Check sheet for the modelled part. Datum: model origin and axes. Units: mm. Coordinates: 2 decimals unless noted, no trailing zeros. Loops run counter-clockwise (first coordinate to the right, second up) from the corner with the lowest first, then second, coordinate; pieces in that order, holes last. Notation, with made-up numbers: (87.25, -1) - (91.25, -1) arc R6 cw to (91.25, 10) - close; hole circle Ø7 at (-22.5, -34.75). An arc over 180 degrees is marked (long way). Answer as a JSON object with one key per item and string values. Group by question number.
from build123d import *

# Parameters (mm, degrees)
RESSALTO_EXTRUS_O1_DEPTH = 2
CORTE_EXTRUS_O1_DEPTH    = 3


with BuildPart() as part:
    # Esboço1 → Ressalto-extrusão1 (new body)
    with BuildSketch(Plane(origin=(0, 0, 0), x_dir=(1, 0, 0), z_dir=(0, 1, 0))):
        with BuildLine():
            Line((-65, 27.690493718), (-17.774626759, 33.612777476))
            ThreePointArc((-17.774626759, 33.612777476), (-17.153688565, 33.671045747), (-16.530325742, 33.690493718))
            Line((-16.530325742, 33.690493718), (0, 33.690493718))
            Line((0, 33.690493718), (0, -23.309506282))
            Line((0, -23.309506282), (-24.541301383, -23.309506282))
            ThreePointArc((-24.541301383, -23.309506282), (-27.628384162, -22.821073972), (-30.413900746, -21.403490265))
            Line((-30.413900746, -21.403490265), (-65, 3.690493718))
            Line((-65, 3.690493718), (-65, 8.690493718))
            Line((-65, 8.690493718), (-67.5, 8.690493718))
            Line((-67.5, 8.690493718), (-67.5, 22.690493718))
            Line((-67.5, 22.690493718), (-65, 22.690493718))
            Line((-65, 22.690493718), (-65, 27.690493718))
        make_face()
    ressalto_extrus_o1 = extrude(amount=RESSALTO_EXTRUS_O1_DEPTH)

    # Espelhar1: Ressalto-extrusão1 across plane
    add(ressalto_extrus_o1.mirror(Plane(origin=(0, 2, 23.309506282), x_dir=(0, 0, 1), z_dir=(-1, 0, 0))))

    # Esboço2 → Corte-extrusão1 (cut, through all)
    with BuildSketch(Plane(origin=(0, 2, 0), x_dir=(1, 0, 0), z_dir=(0, 1, 0))):
        with BuildLine():
            Line((-52.5, 18.690493718), (52.5, 18.690493718))
            ThreePointArc((52.5, 18.690493718), (53.207106781, 18.397600499), (53.5, 17.690493718))
            Line((53.5, 17.690493718), (53.5, 13.190493718))
            ThreePointArc((53.5, 13.190493718), (53.207106781, 12.483386937), (52.5, 12.190493718))
            Line((52.5, 12.190493718), (-7, 12.190493718))
            Line((-7, 12.190493718), (-7, -16.809506282))
            Line((-7, -16.809506282), (-13.5, -16.809506282))
            Line((-13.5, -16.809506282), (-13.5, 12.190493718))
            Line((-13.5, 12.190493718), (-52.5, 12.190493718))
            ThreePointArc((-52.5, 12.190493718), (-53.207106781, 12.483386937), (-53.5, 13.190493718))
            Line((-53.5, 13.190493718), (-53.5, 17.690493718))
            ThreePointArc((-53.5, 17.690493718), (-53.207106781, 18.397600499), (-52.5, 18.690493718))
        make_face()
    extrude(amount=-CORTE_EXTRUS_O1_DEPTH, mode=Mode.SUBTRACT)


solid = part.part
1. Material ranges on line 1 (X direction, y = 1.7, z = -16); line 2 (X direction, y = 1.4, z = -5); line 3 (Z direction, x = -9, y = 0.6), recorded low to high.
2. Sectioned sample at B-B on x = 44.5. Record the cut outline in (y, z), plus the area to 3 significant figures.
3. Gauge pin test, flat ends, axial feed: pin 1 (0.6 mm diameter, centred on x = 66.5, y = 1.5, fed in from +Z); pin 2 (0.6 mm diameter, centred on y = 1, z = -26.5, fed in from +X); pin 3 (0.6 mm diameter, centred on x = 20, y = 1, fed in from -Z). Record the tip position at first contact, or that the pin passes through.
4. Sectioned sample at C-C on z = 11.5. Record the cut outline in (x, y).
5. Sectioned sample at D-D on z = 18.5. Record the cut outline in (x, y).
Answers follow:
{
 "1": {"line 1": "x = -67.5 to -53.5, 53.5 to 67.5", "line 2": "x = -65 to -13.5, -7 to 65", "line 3": "z = -33.69 to -18.69, 16.81 to 23.31"},
 "2": {"outline": "(0, -30.26) - (2, -30.26) - (2, -18.69) - (0, -18.69) - close; (0, -12.19) - (2, -12.19) - (2, 11.18) - (0, 11.18) - close", "area": "69.9 mm^2"},
 "3": {"pin 1": "stops at z = -8.69", "pin 2": "stops at x = 65", "pin 3": "stops at z = -33.37"},
 "4": {"outline": "(-44.06, 0) - (-13.5, 0) - (-13.5, 2) - (-44.06, 2) - close; (-7, 0) - (44.06, 0) - (44.06, 2) - (-7, 2) - close"},
 "5": {"outline": "(-34.42, 0) - (34.42, 0) - (34.42, 2) - (-34.42, 2) - close"}
}
